```python
from build123d import *

# Parameters (mm, degrees)
F0_W     = 30
F0_H     = 6
F3_DEPTH = 7


with BuildPart() as f1:
    # F0 (on Front) → F1 (revolve)
    with BuildSketch(Plane.XZ):
        with Locations((15, 3)):
            Rectangle(F0_W, F0_H)
    revolve(axis=Axis((15, 0, 0), (1, 0, 0)))

    # F2 (on face) → F3 (join)
    with BuildSketch(Plane(origin=(0, 0, 0), x_dir=(0, -1, 0), z_dir=(-1, 0, 0))):
        Polygon((10.962513, -0.395784), (5.824015, 9.295923), (-5.138498, 9.691706), (-10.962513, 0.395784), (-5.824015, -9.295923), (5.138498, -9.691706), align=None)
    extrude(amount=F3_DEPTH)


solid = f1.part
```
The listing builds one solid part. Answer for the finished solid, in the listing's coordinates (mm). A direction names the side the tool comes from. Give positions to 0.01 mm unless a question says otherwise; leave off trailing zeros. Write each loop counter-clockwise with the first axis right and the second up, starting at its lowest first coordinate (ties: lowest second). Pieces come first, ordered by that corner, then holes. Notation, with made-up numbers: (19.25, 2) -> (57.25, 2) arc R15 cw to (57.25, 12) -> close; hole circle Ø6 at (-39.5, 3). An arc over 180 degrees is marked (long way). Use one line per item in the form item = value.
1) A tool of negligible diameter and unlimited length cuts with its end or side. For faces 1 (the flat face through (0, -5, -4)), 2 (the flat face through (-3.45, 8.01, 5.11)), from which of +Z, -Z, +X, -X, +Y, -Y can it reach the whole face along a straight path? Write none if from no direction.
Result:
face_1 = +X
face_2 = +Z, +X, -X, +Y
2) Straight lines are drawn through the part: probe 1 along X at (y, z) = (-7, 0.25); probe 2 along Y at (x, z) = (-3.5, -4.5); probe 3 along Z at (x, y) = (2, 1). For each, find the intervals that lie inside material, in ascending order.
Result:
probe_1 = -7 to 0
probe_2 = -8.39 to 8.37
probe_3 = -5.92 to 5.92
3) Section A-A on x = -0.5 is taken. Write down the section's boundary in (y, z), plus the area to 3 significant figures.
Result:
outline = (-10.96, -0.4) -> (-5.14, -9.69) -> (5.82, -9.3) -> (10.96, 0.4) -> (5.14, 9.69) -> (-5.82, 9.3) -> close
area = 313 mm²
4) Section D-D on x = 4 is taken. Write down the section's boundary in (y, z).
Result:
outline = circle Ø12 at (0, 0)
5) Each of these flat-tipped pins is pushed along its axis until it touches: P1, Ø2, axis at y = -5.5, z = -7, coming from the +X side; P2, Ø3, axis at x = -2, z = -2, coming from the -Y side; P3, Ø8, axis at x = 23, z = -1, coming from the +Y side. Where does it stop, or does it pass through?
Result:
P1 = 0
P2 = -10.9
P3 = 6
6) Section C-C on y = 1.5 is taken. Write down the section's boundary in (x, z).
Result:
outline = (-7, -9.45) -> (0, -9.45) -> (0, -5.81) -> (30, -5.81) -> (30, 5.81) -> (0, 5.81) -> (0, 9.56) -> (-7, 9.56) -> close
7) Section B-B on z = -1.25 is taken. Write down the section's boundary in (x, y), plus the area to 3 significant figures.
Result:
outline = (-7, -10.43) -> (0, -10.43) -> (0, -5.87) -> (30, -5.87) -> (30, 5.87) -> (0, 5.87) -> (0, 10.09) -> (-7, 10.09) -> close
area = 496 mm²
